The model under review builds one solid part; all positions refer to its coordinate system, in mm. Face numbers are marked on the shaded views. Round coordinates to 2 decimals unless told otherwise and drop trailing zeros. Order: outer loops, then holes, each group sorted by start corner. A loop starts at its lowest first (then second) coordinate and runs counter-clockwise, first axis right, second up. Notation, with made-up numbers: (43.5, -29.75) -> (74.5, -29.75) arc R23 cw to (74.5, -12.75) -> close; hole circle Ø6 at (59.5, 73.5). An arc over 180 degrees is marked (long way). Use a Markdown table: item, result. Add a question column.
```python
from build123d import *

# Parameters (mm, degrees)
F0_R     = 0.585
F1_DEPTH = 9.3
F2_DEPTH = 1
F3_DEPTH = 8.3
F4_R     = 0.45
F5_DEPTH = 9.301


with BuildPart() as f1:
    # F0 (on Top) → F1 (new body)
    with BuildSketch(Plane.XY):
        with BuildLine():
            Line((0, 1.21), (-4.8, 1.21))
            ThreePointArc((-4.8, 1.21), (-5.405059, 1.047857), (-5.847959, 0.604882))
            Line((-5.847959, 0.604882), (-7.447959, -2.167118))
            ThreePointArc((-7.447959, -2.167118), (-7.61, -2.772), (-7.447959, -3.376882))
            Line((-7.447959, -3.376882), (-6.647959, -4.762882))
            ThreePointArc((-6.647959, -4.762882), (-6.205059, -5.205857), (-5.6, -5.368))
            Line((-5.6, -5.368), (-0.8, -5.368))
            ThreePointArc((-0.8, -5.368), (-0.194941, -5.205857), (0.247959, -4.762882))
            Line((0.247959, -4.762882), (1.047959, -3.376882))
            ThreePointArc((1.047959, -3.376882), (1.168788, -3.085105), (1.21, -2.772))
            Line((1.21, -2.772), (1.21, 0))
            ThreePointArc((1.21, 0), (0.855599, 0.855599), (0, 1.21))
        make_face()
        with BuildLine():
            ThreePointArc((-5.414918, 0.354931), (-5.155035, 0.614858), (-4.8, 0.71))
            Line((-4.8, 0.71), (0, 0.71))
            ThreePointArc((0, 0.71), (0.502046, 0.502046), (0.71, 0))
            Line((0.71, 0), (0.71, -2.772))
            ThreePointArc((0.71, -2.772), (0.685818, -2.955723), (0.614918, -3.126931))
            Line((0.614918, -3.126931), (-0.185082, -4.512931))
            ThreePointArc((-0.185082, -4.512931), (-0.444965, -4.772858), (-0.8, -4.868))
            Line((-0.8, -4.868), (-5.6, -4.868))
            ThreePointArc((-5.6, -4.868), (-5.955035, -4.772858), (-6.214918, -4.512931))
            Line((-6.214918, -4.512931), (-7.014918, -3.126931))
            ThreePointArc((-7.014918, -3.126931), (-7.11, -2.772), (-7.014918, -2.417069))
            Line((-7.014918, -2.417069), (-5.414918, 0.354931))
        make_face(mode=Mode.SUBTRACT)
        with BuildLine():
            Line((0, 0.71), (-4.8, 0.71))
            ThreePointArc((-4.8, 0.71), (-5.155035, 0.614858), (-5.414918, 0.354931))
            Line((-5.414918, 0.354931), (-7.014918, -2.417069))
            ThreePointArc((-7.014918, -2.417069), (-7.11, -2.772), (-7.014918, -3.126931))
            Line((-7.014918, -3.126931), (-6.214918, -4.512931))
            ThreePointArc((-6.214918, -4.512931), (-5.955035, -4.772858), (-5.6, -4.868))
            Line((-5.6, -4.868), (-0.8, -4.868))
            ThreePointArc((-0.8, -4.868), (-0.444965, -4.772858), (-0.185082, -4.512931))
            Line((-0.185082, -4.512931), (0.614918, -3.126931))
            ThreePointArc((0.614918, -3.126931), (0.685818, -2.955723), (0.71, -2.772))
            Line((0.71, -2.772), (0.71, 0))
            ThreePointArc((0.71, 0), (0.502046, 0.502046), (0, 0.71))
        make_face()
        with Locations((-5.6, -4.158)):
            Circle(F0_R, mode=Mode.SUBTRACT)
        with Locations((-4, -4.158)):
            Circle(F0_R, mode=Mode.SUBTRACT)
        with Locations((-6.4, -2.772)):
            Circle(F0_R, mode=Mode.SUBTRACT)
        with Locations((-4.8, -2.772)):
            Circle(F0_R, mode=Mode.SUBTRACT)
        with Locations((-2.4, -4.158)):
            Circle(F0_R, mode=Mode.SUBTRACT)
        with Locations((-0.8, -4.158)):
            Circle(F0_R, mode=Mode.SUBTRACT)
        with Locations((-3.2, -2.772)):
            Circle(F0_R, mode=Mode.SUBTRACT)
        with Locations((-1.6, -2.772)):
            Circle(F0_R, mode=Mode.SUBTRACT)
        with Locations((0, -2.772)):
            Circle(F0_R, mode=Mode.SUBTRACT)
        with Locations((-5.6, -1.386)):
            Circle(F0_R, mode=Mode.SUBTRACT)
        with Locations((-4, -1.386)):
            Circle(F0_R, mode=Mode.SUBTRACT)
        with Locations((-4.8, 0)):
            Circle(F0_R, mode=Mode.SUBTRACT)
        with Locations((-2.4, -1.386)):
            Circle(F0_R, mode=Mode.SUBTRACT)
        with Locations((-0.8, -1.386)):
            Circle(F0_R, mode=Mode.SUBTRACT)
        with Locations((-3.2, 0)):
            Circle(F0_R, mode=Mode.SUBTRACT)
        with Locations((-1.6, 0)):
            Circle(F0_R, mode=Mode.SUBTRACT)
        Circle(F0_R, mode=Mode.SUBTRACT)
        with Locations((-0.8, -4.158)):
            Circle(F0_R)
        with Locations((0, -2.772)):
            Circle(F0_R)
        with Locations((-0.8, -1.386)):
            Circle(F0_R)
        Circle(F0_R)
        with Locations((-1.6, 0)):
            Circle(F0_R)
        with Locations((-3.2, 0)):
            Circle(F0_R)
        with Locations((-4.8, 0)):
            Circle(F0_R)
        with Locations((-5.6, -1.386)):
            Circle(F0_R)
        with Locations((-4, -1.386)):
            Circle(F0_R)
        with Locations((-2.4, -1.386)):
            Circle(F0_R)
        with Locations((-1.6, -2.772)):
            Circle(F0_R)
        with Locations((-3.2, -2.772)):
            Circle(F0_R)
        with Locations((-6.4, -2.772)):
            Circle(F0_R)
        with Locations((-5.6, -4.158)):
            Circle(F0_R)
        with Locations((-4, -4.158)):
            Circle(F0_R)
        with Locations((-2.4, -4.158)):
            Circle(F0_R)
        with Locations((-4.8, -2.772)):
            Circle(F0_R)
    extrude(amount=-F1_DEPTH)

    # F0 (on Top) → F2 (cut)
    with BuildSketch(Plane.XY):
        with BuildLine():
            Line((0, 0.71), (-4.8, 0.71))
            ThreePointArc((-4.8, 0.71), (-5.155035, 0.614858), (-5.414918, 0.354931))
            Line((-5.414918, 0.354931), (-7.014918, -2.417069))
            ThreePointArc((-7.014918, -2.417069), (-7.11, -2.772), (-7.014918, -3.126931))
            Line((-7.014918, -3.126931), (-6.214918, -4.512931))
            ThreePointArc((-6.214918, -4.512931), (-5.955035, -4.772858), (-5.6, -4.868))
            Line((-5.6, -4.868), (-0.8, -4.868))
            ThreePointArc((-0.8, -4.868), (-0.444965, -4.772858), (-0.185082, -4.512931))
            Line((-0.185082, -4.512931), (0.614918, -3.126931))
            ThreePointArc((0.614918, -3.126931), (0.685818, -2.955723), (0.71, -2.772))
            Line((0.71, -2.772), (0.71, 0))
            ThreePointArc((0.71, 0), (0.502046, 0.502046), (0, 0.71))
        make_face()
        with Locations((-5.6, -4.158)):
            Circle(F0_R, mode=Mode.SUBTRACT)
        with Locations((-4, -4.158)):
            Circle(F0_R, mode=Mode.SUBTRACT)
        with Locations((-6.4, -2.772)):
            Circle(F0_R, mode=Mode.SUBTRACT)
        with Locations((-4.8, -2.772)):
            Circle(F0_R, mode=Mode.SUBTRACT)
        with Locations((-2.4, -4.158)):
            Circle(F0_R, mode=Mode.SUBTRACT)
        with Locations((-0.8, -4.158)):
            Circle(F0_R, mode=Mode.SUBTRACT)
        with Locations((-3.2, -2.772)):
            Circle(F0_R, mode=Mode.SUBTRACT)
        with Locations((-1.6, -2.772)):
            Circle(F0_R, mode=Mode.SUBTRACT)
        with Locations((0, -2.772)):
            Circle(F0_R, mode=Mode.SUBTRACT)
        with Locations((-5.6, -1.386)):
            Circle(F0_R, mode=Mode.SUBTRACT)
        with Locations((-4, -1.386)):
            Circle(F0_R, mode=Mode.SUBTRACT)
        with Locations((-4.8, 0)):
            Circle(F0_R, mode=Mode.SUBTRACT)
        with Locations((-2.4, -1.386)):
            Circle(F0_R, mode=Mode.SUBTRACT)
        with Locations((-0.8, -1.386)):
            Circle(F0_R, mode=Mode.SUBTRACT)
        with Locations((-3.2, 0)):
            Circle(F0_R, mode=Mode.SUBTRACT)
        with Locations((-1.6, 0)):
            Circle(F0_R, mode=Mode.SUBTRACT)
        Circle(F0_R, mode=Mode.SUBTRACT)
        with Locations((-4.8, 0)):
            Circle(F0_R)
        with Locations((-5.6, -1.386)):
            Circle(F0_R)
        with Locations((-6.4, -2.772)):
            Circle(F0_R)
        with Locations((-5.6, -4.158)):
            Circle(F0_R)
        with Locations((-4.8, -2.772)):
            Circle(F0_R)
        with Locations((-4, -4.158)):
            Circle(F0_R)
        with Locations((-4, -1.386)):
            Circle(F0_R)
        with Locations((-3.2, 0)):
            Circle(F0_R)
        with Locations((-1.6, 0)):
            Circle(F0_R)
        with Locations((-2.4, -1.386)):
            Circle(F0_R)
        with Locations((-3.2, -2.772)):
            Circle(F0_R)
        with Locations((-2.4, -4.158)):
            Circle(F0_R)
        Circle(F0_R)
        with Locations((-0.8, -1.386)):
            Circle(F0_R)
        with Locations((-1.6, -2.772)):
            Circle(F0_R)
        with Locations((-0.8, -4.158)):
            Circle(F0_R)
        with Locations((0, -2.772)):
            Circle(F0_R)
    extrude(amount=-F2_DEPTH, mode=Mode.SUBTRACT)

    # F0 (on Top) → F3 (cut)
    with BuildSketch(Plane.XY):
        with Locations((-6.4, -2.772)):
            Circle(F0_R)
        with Locations((-5.6, -1.386)):
            Circle(F0_R)
        with Locations((-4.8, 0)):
            Circle(F0_R)
        with Locations((-5.6, -4.158)):
            Circle(F0_R)
        with Locations((-4.8, -2.772)):
            Circle(F0_R)
        with Locations((-4, -1.386)):
            Circle(F0_R)
        with Locations((-3.2, 0)):
            Circle(F0_R)
        with Locations((-1.6, 0)):
            Circle(F0_R)
        with Locations((-2.4, -1.386)):
            Circle(F0_R)
        with Locations((-3.2, -2.772)):
            Circle(F0_R)
        with Locations((-4, -4.158)):
            Circle(F0_R)
        with Locations((-2.4, -4.158)):
            Circle(F0_R)
        with Locations((-1.6, -2.772)):
            Circle(F0_R)
        with Locations((-0.8, -1.386)):
            Circle(F0_R)
        Circle(F0_R)
        with Locations((0, -2.772)):
            Circle(F0_R)
        with Locations((-0.8, -4.158)):
            Circle(F0_R)
    extrude(amount=-F3_DEPTH, mode=Mode.SUBTRACT)

    # F4 (on Top) → F5 (cut, through all)
    with BuildSketch(Plane.XY):
        with Locations((-4.8, 0)):
            Circle(F4_R)
        with Locations((-3.2, 0)):
            Circle(F4_R)
        with Locations((-1.6, 0)):
            Circle(F4_R)
        Circle(F4_R)
        with Locations((-0.8, -1.386)):
            Circle(F4_R)
        with Locations((-2.4, -1.386)):
            Circle(F4_R)
        with Locations((-4, -1.386)):
            Circle(F4_R)
        with Locations((-5.6, -1.386)):
            Circle(F4_R)
        with Locations((-6.4, -2.772)):
            Circle(F4_R)
        with Locations((-4.8, -2.772)):
            Circle(F4_R)
        with Locations((-3.2, -2.772)):
            Circle(F4_R)
        with Locations((-1.6, -2.772)):
            Circle(F4_R)
        with Locations((0, -2.772)):
            Circle(F4_R)
        with Locations((-0.8, -4.158)):
            Circle(F4_R)
        with Locations((-2.4, -4.158)):
            Circle(F4_R)
        with Locations((-4, -4.158)):
            Circle(F4_R)
        with Locations((-5.6, -4.158)):
            Circle(F4_R)
    extrude(amount=-F5_DEPTH, mode=Mode.SUBTRACT)


solid = f1.part
```
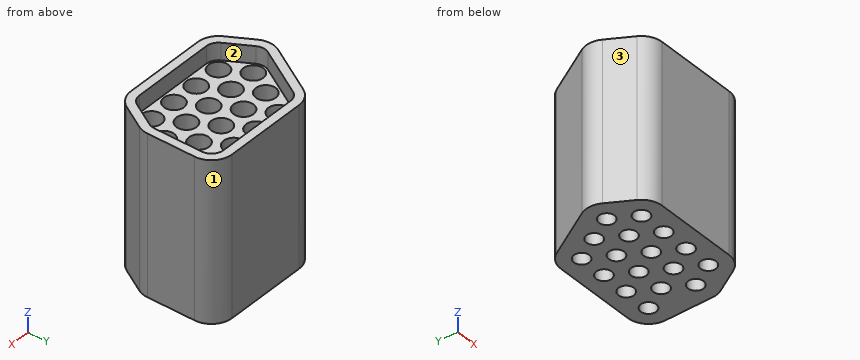
Q1. Add section A-A, the plane x = -1.6. Give the boundary of the cut face in (y, z) (3 decimals).
Q2. Add section C-C, the plane z = -4. Give the number of separate pieces and of enclosed holes in the cut face, then the cut area to 3 significant figures.
Q3. Add section B-B, the plane x = -6.5. Give the boundary of the cut face in (y, z).
Q4. For pin 1 (1.9 mm diameter, centred on x = -0.8, y = -1.386, fed in from +Z); pin 2 (1.1 mm diameter, centred on y = -1.5, z = -0.5, fed in from -X), all flat-tipped, find the tip position at first contact; note any pin that passes through.
Q5. To check wall thickness, follow line 1 along X through (y, z) = (0.5, -1.5); line 2 along Y through (x, z) = (-2.4, -8.8); line 3 along Y through (x, z) = (-1.75, -2). State the ranges of each line that lie inside material, in increasing order.
Q6. Draft analysis for pull direction X (two halves, no side actions). For the marked faces 1, 2 and 3, state which applies: released by +X, released by -X, zero draft, split by the parting line, or undercut.
Return value:
| question | item | result |
|---|---|---|
| 1 | outline | (-5.368, -9.3) -> (-3.222, -9.3) -> (-3.222, -8.3) -> (-3.357, -8.3) -> (-3.357, -1) -> (-4.868, -1) -> (-4.868, 0) -> (-5.368, 0) -> close; (-2.322, -9.3) -> (-0.45, -9.3) -> (-0.45, -8.3) -> (-0.585, -8.3) -> (-0.585, -1) -> (-2.187, -1) -> (-2.187, -8.3) -> (-2.322, -8.3) -> close; (0.45, -9.3) -> (1.21, -9.3) -> (1.21, 0) -> (0.71, 0) -> (0.71, -1) -> (0.585, -1) -> (0.585, -8.3) -> (0.45, -8.3) -> close |
| 2 | separate pieces | 1 |
| 2 | enclosed holes | 17 |
| 2 | area | 32.3 mm² |
| 3 | outline | (-4.97, -9.3) -> (-3.21, -9.3) -> (-3.21, -8.3) -> (-3.35, -8.3) -> (-3.35, -1) -> (-4.02, -1) -> (-4.02, 0) -> (-4.97, 0) -> close; (-2.33, -9.3) -> (-0.52, -9.3) -> (-0.52, 0) -> (-1.52, 0) -> (-1.52, -1) -> (-2.2, -1) -> (-2.2, -8.3) -> (-2.33, -8.3) -> close |
| 4 | pin 1 | z = -1 |
| 4 | pin 2 | x = -7.38 |
| 5 | line 1 | -5.91 to -5.1, -4.5 to -3.5, -2.9 to -1.9, -1.3 to -0.3, 0.3 to 1.1 |
| 5 | line 2 | -5.37 to -4.61, -3.71 to -1.84, -0.94 to 1.21 |
| 5 | line 3 | -5.37 to -3.34, -2.21 to -0.57, 0.57 to 1.21 |
| 6 | face 1 | released by +X |
| 6 | face 2 | undercut |
| 6 | face 3 | released by -X |
